from build123d import *

# Parameters (mm, degrees)
SKETCH173_W     = 24
SKETCH173_H     = 10.4
PAD043_DEPTH    = 30
SKETCH174_W     = 24
SKETCH174_H     = 10.4
PAD044_DEPTH    = 8
SKETCH175_R     = 2.75
POCKET095_DEPTH = 8
SKETCH176_R     = 5.25
POCKET096_DEPTH = 3
SKETCH177_R     = 2.55
POCKET097_DEPTH = 36.551
CHAMFER072_SIZE = 3
FILLET045_R     = 2
CHAMFER073_SIZE = 1.5


with BuildPart() as part:
    # Sketch173 → Pad043 (new body)
    with BuildSketch(Plane.XY):
        Polygon((-18, 36.55), (18, 36.55), (18, 32.55), (16, 32.55), (16, 22.15), (32, 22.15), (32, 18.15), (-32, 18.15), (-32, 22.15), (-16, 22.15), (-16, 32.55), (-18, 32.55), align=None)
        with Locations((0, 27.35)):
            Rectangle(SKETCH173_W, SKETCH173_H, mode=Mode.SUBTRACT)
    extrude(amount=PAD043_DEPTH)

    # Sketch174 → Pad044 (join)
    with BuildSketch(Plane.XY):
        with Locations((0, 27.35)):
            Rectangle(SKETCH174_W, SKETCH174_H)
    extrude(amount=PAD044_DEPTH)

    # Sketch175 → Pocket095 (cut)
    with BuildSketch(Plane.XY):
        with Locations((0, 27.35)):
            Circle(SKETCH175_R)
    extrude(amount=POCKET095_DEPTH, mode=Mode.SUBTRACT)

    # Sketch176 → Pocket096 (cut)
    with BuildSketch(Plane.XY.offset(8)):
        with Locations((0, 27.35)):
            Circle(SKETCH176_R)
    extrude(amount=-POCKET096_DEPTH, mode=Mode.SUBTRACT)

    # Sketch177 → Pocket097 (cut, through all)
    with BuildSketch(Plane.XZ):
        with Locations((0, 18)):
            Circle(SKETCH177_R)
    extrude(amount=-POCKET097_DEPTH, mode=Mode.SUBTRACT)

    # Chamfer072
    chamfer072_edges = [part.edges().sort_by_distance(p)[0] for p in [
        (-16, 22.15, 15),
        (16, 22.15, 15),
    ]]
    chamfer(chamfer072_edges, length=CHAMFER072_SIZE)

    # Fillet045
    fillet045_edges = [part.edges().sort_by_distance(p)[0] for p in [
        (-18, 36.55, 15),
        (18, 36.55, 15),
        (-32, 18.15, 15),
        (32, 18.15, 15),
    ]]
    fillet(fillet045_edges, radius=FILLET045_R)

    # Chamfer073
    chamfer073_edges = [part.edges().sort_by_distance(p)[0] for p in [
        (-16, 32.55, 15),
        (16, 32.55, 15),
    ]]
    chamfer(chamfer073_edges, length=CHAMFER073_SIZE)


solid = part.part
CAD build for the part. Positions are in the model's coordinates, mm. A direction names the side the tool comes from. Coordinates: 2 decimals unless noted, no trailing zeros. Write each loop counter-clockwise with the first axis right and the second up, starting at its lowest first coordinate (ties: lowest second). Pieces come first, ordered by that corner, then holes. Notation, with made-up numbers: M 43.25,-7.5 L 48.25,-7.5 A17 ccw 48.25,8.5 Z; hole C 37,-3.5 d11. An arc over 180 degrees is marked long. Answer as a JSON object with one key per item and string values. Group by question number.
1) Saw through at A-A (y = 27.35). Write the cut outline in (x, z), plus the area to 3 significant figures.
2) Pin check, flat tips, straight feed: pin 1 Ø6 at (x, z) = (0, 18) entering from -Y; pin 2 Ø4.5 at (y, z) = (27.5, 21.5) entering from +X; pin 3 Ø2 at (y, z) = (33.5, 19) entering from -X; pin 4 Ø5 at (x, y) = (-8.5, 29.5) entering from +Z. Stop position of each tip, or through.
3) Saw through at C-C (x = 0). Write the cut outline in (y, z), plus the area to 3 significant figures.
4) Wall check: line 1 (Y direction, x = 0, z = 3); line 2 (X direction, y = 27.35, z = 6.6); line 3 (Y direction, x = -10.5, z = 13.5). Give the ranges that are in metal, low to high. Write a range as from..to.
5) Tool access for faces 4 (the face through (17.52, 23.63, 14.79)), 5 (the face through (-18, 34, 15)), 6 (the face through (-12, 27, 19)): list every direction of +Z, -Z, +X, -X, +Y, -Y with a clear straight run to the whole face (end or side of a thin tool).
6) Saw through at D-D (z = 14). Write the cut outline in (x, y), plus the area to 3 significant figures.
7) Mould opens along X. For faces 1 (the face through (-16.74, 31.79, 14.79)), 2 (the face through (2, 25, 5)), 3 (the face through (16.74, 31.79, 14.79)) say: +X half, -X half, draft (parallel to the pull), parting line (faces both ways), or undercut.
Values follow:
{
 "1": {"outline": "M -16,0 L -2.75,0 L -2.75,5 L -5.25,5 L -5.25,8 L -12,8 L -12,30 L -16,30 Z; M 2.75,0 L 16,0 L 16,30 L 12,30 L 12,8 L 5.25,8 L 5.25,5 L 2.75,5 Z", "area": "373 mm2"},
 "2": {"pin 1": "stops at y = 18.15", "pin 2": "stops at x = 16", "pin 3": "stops at x = -18", "pin 4": "stops at z = 8"},
 "3": {"outline": "M 18.15,0 L 24.6,0 L 24.6,5 L 22.1,5 L 22.1,8 L 22.15,8 L 22.15,15.45 L 18.15,15.45 Z; M 18.15,20.55 L 22.15,20.55 L 22.15,30 L 18.15,30 Z; M 30.1,0 L 36.55,0 L 36.55,15.45 L 32.55,15.45 L 32.55,8 L 32.6,8 L 32.6,5 L 30.1,5 Z; M 32.55,20.55 L 36.55,20.55 L 36.55,30 L 32.55,30 Z", "area": "223 mm2"},
 "4": {"line 1": "y = 18.15..24.6, 30.1..36.55", "line 2": "x = -16..-5.25, 5.25..16", "line 3": "y = 18.15..22.15, 32.55..36.55"},
 "5": {"face 4": "+Z, -Z, +X", "face 5": "+Z, -Z, -X, +Y", "face 6": "+Z"},
 "6": {"outline": "M -32,20.15 A2 ccw -30,18.15 L 30,18.15 A2 ccw 32,20.15 L 32,22.15 L 19,22.15 L 16,25.15 L 16,31.05 L 17.5,32.55 L 18,32.55 L 18,34.55 A2 ccw 16,36.55 L -16,36.55 A2 ccw -18,34.55 L -18,32.55 L -17.5,32.55 L -16,31.05 L -16,25.15 L -19,22.15 L -32,22.15 Z; hole M -12,22.15 L 12,22.15 L 12,32.55 L -12,32.55 Z", "area": "491 mm2"},
 "7": {"face 1": "-X half", "face 2": "undercut", "face 3": "+X half"}
}
